from build123d import *

# Parameters (mm, degrees)
SKETCH_1_W          = 59
SKETCH_1_H          = 51
EXTRUDE_1_DEPTH     = 10
CUT_EXTRUDE_1_DEPTH = 5
CUT_EXTRUDE_2_DEPTH = 5
HOLE_WIZARD_M31_D   = 3.4
FILLET_1_R          = 4
FILLET_2_R          = 4
HOLE_WIZARD_M41_D   = 4.5
CUT_EXTRUDE_4_DEPTH = 5


with BuildPart() as part:
    # Эскиз1 → Бобышка-Вытянуть1 (new body)
    with BuildSketch(Plane(origin=(0, 0, 0), x_dir=(1, 0, 0), z_dir=(0, 1, 0))):
        with Locations((29.5, 25.5)):
            Rectangle(SKETCH_1_W, SKETCH_1_H)
    extrude(amount=EXTRUDE_1_DEPTH)

    # Эскиз3 → Вырез-Вытянуть1 (cut)
    with BuildSketch(Plane(origin=(28.521351565, 10, -17.681729678), x_dir=(1, 0, 0), z_dir=(0, 1, 0))):
        with BuildLine():
            Line((-23.621351565, -11.07668717), (-23.621351565, -17.781729678))
            Line((-23.621351565, -17.781729678), (6.578648435, -17.781729678))
            Line((6.578648435, -17.781729678), (6.578648435, -11.07668717))
            ThreePointArc((6.578648435, -11.07668717), (6.552127505, -10.672055974), (6.473018496, -10.27434813))
            Line((6.473018496, -10.27434813), (5.027443993, -4.879390638))
            ThreePointArc((5.027443993, -4.879390638), (3.920234361, -3.222334323), (2.033073931, -2.581729678))
            Line((2.033073931, -2.581729678), (-19.075777062, -2.581729678))
            ThreePointArc((-19.075777062, -2.581729678), (-20.962937492, -3.222334323), (-22.070147123, -4.879390638))
            Line((-22.070147123, -4.879390638), (-23.515721627, -10.27434813))
            ThreePointArc((-23.515721627, -10.27434813), (-23.594830635, -10.672055974), (-23.621351565, -11.07668717))
        make_face()
    extrude(amount=-CUT_EXTRUDE_1_DEPTH, mode=Mode.SUBTRACT)

    # Эскиз4 → Вырез-Вытянуть2 (cut)
    with BuildSketch(Plane(origin=(0, 10, 0), x_dir=(1, 0, 0), z_dir=(0, 1, 0))):
        with BuildLine():
            Line((-1.551204442, 38.19766096), (-0.105629939, 43.592618453))
            ThreePointArc((-0.105629939, 43.592618453), (-0.02652093, 43.990326297), (0, 44.394957493))
            Line((0, 44.394957493), (0, 51))
            Line((0, 51), (-30.2, 51))
            Line((-30.2, 51), (-30.2, 44.394957493))
            ThreePointArc((-30.2, 44.394957493), (-30.17347907, 43.990326297), (-30.094370061, 43.592618453))
            Line((-30.094370061, 43.592618453), (-28.648795558, 38.19766096))
            ThreePointArc((-28.648795558, 38.19766096), (-27.541585927, 36.540604645), (-25.654425497, 35.9))
            Line((-25.654425497, 35.9), (-4.545574503, 35.9))
            ThreePointArc((-4.545574503, 35.9), (-2.658414073, 36.540604645), (-1.551204442, 38.19766096))
        make_face()
        with BuildLine():
            Line((46.19766096, 11.951204442), (51.592618453, 10.505629939))
            ThreePointArc((51.592618453, 10.505629939), (51.990326297, 10.42652093), (52.394957493, 10.4))
            Line((52.394957493, 10.4), (59, 10.4))
            Line((59, 10.4), (59, 40.6))
            Line((59, 40.6), (52.394957493, 40.6))
            ThreePointArc((52.394957493, 40.6), (51.990326297, 40.57347907), (51.592618453, 40.494370061))
            Line((51.592618453, 40.494370061), (46.19766096, 39.048795558))
            ThreePointArc((46.19766096, 39.048795558), (44.540604645, 37.941585927), (43.9, 36.054425497))
            Line((43.9, 36.054425497), (43.9, 14.945574503))
            ThreePointArc((43.9, 14.945574503), (44.540604645, 13.058414073), (46.19766096, 11.951204442))
        make_face()
    extrude(amount=-CUT_EXTRUDE_2_DEPTH, mode=Mode.SUBTRACT)

    # Отверстие с зазором M31 (through all)
    with Locations(Plane(origin=(0, 0, 0), x_dir=(-1, 0, 0), z_dir=(0, -1, 0))):
        with Locations((-24.242640687, 29.742640687), (-15.757359313, 29.742640687), (-15.757359313, 21.257359313), (-24.242640687, 21.257359313)):
            Hole(HOLE_WIZARD_M31_D / 2)

    # Скругление1
    fillet_1_edges = [part.edges().sort_by_distance(p)[0] for p in [
        (0, 5, -51),
        (0, 5, 0),
    ]]
    fillet(fillet_1_edges, radius=FILLET_1_R)

    # Скругление2
    fillet_2_edges = [part.edges().sort_by_distance(p)[0] for p in [
        (59, 5, -51),
        (59, 5, 0),
    ]]
    fillet(fillet_2_edges, radius=FILLET_2_R)

    # Отверстие с зазором M41 (through all)
    with Locations(Plane(origin=(0, 0, 0), x_dir=(-1, 0, 0), z_dir=(0, -1, 0))):
        with Locations((-51.5, 25.5), (-20, 43.5), (-20, 7.5)):
            Hole(HOLE_WIZARD_M41_D / 2)

    # Эскиз12 → Вырез-Вытянуть4 (cut)
    with BuildSketch(Plane(origin=(0, 10, 0), x_dir=(1, 0, 0), z_dir=(0, 1, 0))):
        with BuildLine():
            Line((4.9, 44.394957493), (4.9, 51))
            Line((4.9, 51), (35.1, 51))
            Line((35.1, 51), (35.1, 44.394957493))
            ThreePointArc((35.1, 44.394957493), (35.07347907, 43.990326297), (34.994370061, 43.592618453))
            Line((34.994370061, 43.592618453), (33.548795558, 38.19766096))
            ThreePointArc((33.548795558, 38.19766096), (32.441585927, 36.540604645), (30.554425497, 35.9))
            Line((30.554425497, 35.9), (9.445574503, 35.9))
            ThreePointArc((9.445574503, 35.9), (7.558414073, 36.540604645), (6.451204442, 38.19766096))
            Line((6.451204442, 38.19766096), (5.005629939, 43.592618453))
            ThreePointArc((5.005629939, 43.592618453), (4.92652093, 43.990326297), (4.9, 44.394957493))
        make_face()
    extrude(amount=-CUT_EXTRUDE_4_DEPTH, mode=Mode.SUBTRACT)


solid = part.part
Design review of the part built by this model. Coordinates are the model's own, in mm. A direction names the side the tool comes from. Coordinates: 2 decimals unless noted, no trailing zeros. Order: outer loops, then holes, each group sorted by start corner. A loop starts at its lowest first (then second) coordinate and runs counter-clockwise, first axis right, second up. Notation, with made-up numbers: (67, 64.25) -> (71, 64.25) arc R29 ccw to (71, 97.25) -> close; hole circle Ø6 at (-17, 24.5). An arc over 180 degrees is marked (long way). One line per item, written item: value.
1) Clearance check with flat-ended pins moving along their axes: P1, Ø2.5, axis at x = 15.76, z = -29.74, coming from the -Y side; P2, Ø1.5, axis at y = 8, z = -49.5, coming from the -X side; P3, Ø4.5, axis at x = 22, z = -6.5, coming from the +Y side; P4, Ø2.5, axis at x = 57, y = 6.5, coming from the -Z side. State where each tip first meets the part, or that it passes through.
Output values:
P1: passes through
P2: stops at x = 0.4
P3: stops at y = 5
P4: stops at z = -50.93
2) We need section C-C, the plane y = 3.25. Give the boundary of the cut face in (x, z).
Output values:
outline: (0, -47) arc R4 ccw to (4, -51) -> (55, -51) arc R4 ccw to (59, -47) -> (59, -4) arc R4 ccw to (55, 0) -> (4, 0) arc R4 ccw to (0, -4) -> close; hole circle Ø3.4 at (15.76, -29.74); hole circle Ø3.4 at (15.76, -21.26); hole circle Ø4.5 at (20, -43.5); hole circle Ø4.5 at (20, -7.5); hole circle Ø3.4 at (24.24, -29.74); hole circle Ø3.4 at (24.24, -21.26); hole circle Ø4.5 at (51.5, -25.5)
3) We need section D-D, the plane y = 6.5. Count the separate pieces of the cut face and the enclosed holes in it, then the cut area to 3 significant figures.
Output values:
separate pieces: 1
enclosed holes: 4
area: 1,650 mm2
4) We need section A-A, the plane x = 20. Give the boundary of the cut face in (y, z).
Output values:
outline: (0, -51) -> (5, -51) -> (5, -45.75) -> (0, -45.75) -> close; (0, -41.25) -> (5, -41.25) -> (5, -35.9) -> (10, -35.9) -> (10, -15.1) -> (5, -15.1) -> (5, -9.75) -> (0, -9.75) -> close; (0, -5.25) -> (5, -5.25) -> (5, 0) -> (0, 0) -> close
5) To check wall thickness, follow probe 1 along Z at (x, y) = (20, 3.75); probe 2 along Z at (x, y) = (21.5, 3); probe 3 along Z at (x, y) = (51.5, 1.7). State the ranges of each line that lie inside material, in increasing order. Write a range as [from, to].
Output values:
probe 1: z = [-51, -45.75], [-41.25, -9.75], [-5.25, 0]
probe 2: z = [-51, -45.18], [-41.82, -9.18], [-5.82, 0]
probe 3: z = [-51, -27.75], [-23.25, 0]
6) Machinability: for faces 1 (the face through (56, 8, -40.6)), 2 (the face through (4.9, 8, -48)), 3 (the face through (7.581, 7.535, -14.477)), which of the approach directions +Z, -Z, +X, -X, +Y, -Y give a long, thin tool a straight path to every point of the face, cutting with its end or side? Answer none if there is none.
Output values:
face 1: +X, +Y
face 2: -Z, +Y
face 3: +Z, +Y
7) We need section B-B, the plane z = -20.5. Give the boundary of the cut face in (x, y), then the cut area to 3 significant figures.
Output values:
outline: (0, 0) -> (14.24, 0) -> (14.24, 10) -> (0, 10) -> close; (17.28, 0) -> (22.72, 0) -> (22.72, 10) -> (17.28, 10) -> close; (25.76, 0) -> (59, 0) -> (59, 5) -> (43.9, 5) -> (43.9, 10) -> (25.76, 10) -> close
area: 454 mm2
